Can you work these out from the model? Positions are in its coordinate system, mm. A direction names the side the tool comes from. Coordinates: 2 decimals unless noted, no trailing zeros. Write each loop counter-clockwise with the first axis right and the second up, starting at its lowest first coordinate (ties: lowest second). Pieces come first, ordered by that corner, then holes. Notation, with made-up numbers: (48, -3.75) - (100, -3.75) arc R18 cw to (100, 14.25) - close; hole circle Ø1 at (16.5, -30.5). An arc over 180 degrees is marked (long way). Use one line per item in the form item = value. Start each with the question number.
(1) If I drill on probe 1 along Y at (x, z) = (27, 15.5); probe 2 along X at (y, z) = (-23.5, 15); probe 3 along Y at (x, z) = (-36, 15.5), over which ranges is the centre line in solid material (lowest first)? Write a range as from..to.
(2) For pin 1 Ø1.8 at (y, z) = (6, 29) entering from +X; pin 2 Ø6 at (x, z) = (13, 31) entering from +Y; pin 3 Ø1.1 at (y, z) = (-6.5, 26.5) entering from +X, each with a flat end and sliding along its axis, tell me the tip position at first contact or that it passes through.
(3) If we section it at B-B on x = 26: Please give me the cut outline in (y, z).
(4) If we section it at A-A on y = 28: Please give me the cut outline in (x, z), then the cut area to 3 significant figures.
(5) If we section it at D-D on x = -30: Please give me the cut outline in (y, z), then the cut area to 3 significant figures.
(6) If we section it at C-C on z = 16: Please give me the cut outline in (x, y).
(7) On a 3-axis mill with a long thin cutter (end or side, diameter ignored), from which of +Z, -Z, +X, -X, +Y, -Y can I reach the whole of each face in a straight line? I mean faces 1 (the face through (-43, -7.795, 20)), 2 (the face through (-46, 7.795, 22)), 3 (the face through (-41, -55.766, 6)). Say none if no direction works.
```python
from build123d import *

# Parameters (mm, degrees)
F1_DEPTH = 12.7
F0_R     = 40.785869
F2_DEPTH = 38.1
F4_DEPTH = 25.4
F6_DEPTH = 69.326828


with BuildPart() as f1:
    # F0 (on Top) → F1 (new body)
    with BuildSketch(Plane.XY):
        with BuildLine():
            Line((-0.29745, 55.766355), (-80.107197, 55.766355))
            Line((-80.107197, 55.766355), (-80.107197, -55.766355))
            Line((-80.107197, -55.766355), (-0.29745, -55.766355))
            ThreePointArc((-0.29745, -55.766355), (-35.825811, 0), (-0.29745, 55.766355))
        make_face()
    extrude(amount=F1_DEPTH)

    # F0 (on Top) → F2 (join)
    with BuildSketch(Plane.XY):
        with BuildLine():
            ThreePointArc((87.235052, 0), (58.765741, 51.893702), (-0.29745, 55.766355))
            ThreePointArc((-0.29745, 55.766355), (-35.825811, 0), (-0.29745, -55.766355))
            ThreePointArc((-0.29745, -55.766355), (58.765741, -51.893702), (87.235052, 0))
        make_face()
        with Locations((25.70462, 0)):
            Circle(F0_R, mode=Mode.SUBTRACT)
    extrude(amount=F2_DEPTH)

    # F3 (on face) → F4 (join)
    with BuildSketch(Plane.XY.offset(12.7)):
        with BuildLine():
            Line((-35.681184, 7.795396), (-62.072869, 7.795396))
            Line((-62.072869, 7.795396), (-62.072869, -7.795396))
            Line((-62.072869, -7.795396), (-35.681184, -7.795396))
            Line((-35.681184, -7.795396), (-35.681184, -4.216278))
            ThreePointArc((-35.681184, -4.216278), (-35.825811, 0), (-35.681184, 4.216278))
            Line((-35.681184, 4.216278), (-35.681184, 7.795396))
        make_face()
    extrude(amount=F4_DEPTH)

    # F5 (on face) → F6 (cut, through all)
    with BuildSketch(Plane.XZ.offset(7.795396)):
        Polygon((-62.072869, 38.1), (-62.072869, 12.7), (-35.681184, 38.1), align=None)
    extrude(amount=-F6_DEPTH, mode=Mode.SUBTRACT)


solid = f1.part
```
Reported:
q1.probe_1 = -61.52..-40.77, 40.77..61.52
q1.probe_2 = -31.16..-7.63, 59.04..82.57
q1.probe_3 = -7.8..7.8
q2.pin_1 = 87.02
q2.pin_2 = 60.76
q2.pin_3 = 86.95
q3.outline = (-61.53, 0) - (-40.78, 0) - (-40.78, 38.1) - (-61.53, 38.1) - close; (40.78, 0) - (61.53, 0) - (61.53, 38.1) - (40.78, 38.1) - close
q4.outline = (-80.11, 0) - (-3.95, 0) - (-3.95, 38.1) - (-29.09, 38.1) - (-29.09, 12.7) - (-80.11, 12.7) - close; (55.36, 0) - (80.5, 0) - (80.5, 38.1) - (55.36, 38.1) - close
q4.area = 2,560 mm2
q5.outline = (-55.77, 0) - (55.77, 0) - (55.77, 12.7) - (26.13, 12.7) - (26.13, 38.1) - (-26.13, 38.1) - (-26.13, 12.7) - (-55.77, 12.7) - close
q5.area = 2,740 mm2
q6.outline = (-58.64, -7.8) - (-35.68, -7.8) - (-35.68, -4.22) arc R61.53 ccw (long way) to (-35.68, 4.22) - (-35.68, 7.8) - (-58.64, 7.8) - close; hole circle Ø81.57 at (25.7, 0)
q7.face_1 = +Z, -X, -Y
q7.face_2 = +Z, -X, +Y
q7.face_3 = +Z, -Z, -X, -Y
